from build123d import *

# Parameters (mm, degrees)
F1_DEPTH       = 6.22
F2_W           = 7
F2_H           = 1
F3_DEPTH       = 60.201
F4_R           = 0.1
F6_D           = 6.4
F6_CSINK_D     = 13.5
F6_CSINK_ANGLE = 90


with BuildPart() as f1:
    # F0 (on Front) → F1 (new body)
    with BuildSketch(Plane.XZ):
        with BuildLine():
            Line((-53.25, 0), (-0.5, 0))
            ThreePointArc((-0.5, 0), (-0.1464466094, 0.1464466094), (0, 0.5))
            Line((0, 0.5), (0, 59.7))
            ThreePointArc((0, 59.7), (-0.1464466094, 60.0535533906), (-0.5, 60.2))
            Line((-0.5, 60.2), (-53.25, 60.2))
            ThreePointArc((-53.25, 60.2), (-56.7855339059, 58.7355339059), (-58.25, 55.2))
            Line((-58.25, 55.2), (-58.25, 5))
            ThreePointArc((-58.25, 5), (-56.7855339059, 1.4644660941), (-53.25, 0))
        make_face()
    extrude(amount=F1_DEPTH)

    # F2 (on face) → F3 (cut, through all)
    with BuildSketch(Plane.XY.offset(60.2)):
        with Locations((-3.5, -0.5)):
            Rectangle(F2_W, F2_H)
    extrude(amount=-F3_DEPTH, mode=Mode.SUBTRACT)

    # F4
    f4_edges = [f1.edges().sort_by_distance(p)[0] for p in [
        (-26.875, -6.22, 60.2),
        (-30.125, 0, 60.2),
        (-7, 0, 30.1),
        (-3.75, -1, 60.2),
        (-7, -0.5, 60.2),
        (-7, -0.5, 0),
        (-7, -1, 30.1),
    ]]
    fillet(f4_edges, radius=F4_R)

    # F6 (through all)
    with Locations(Plane.XZ.offset(6.22)):
        with Locations((-30.25, 46.05), (-30.25, 14.15)):
            CounterSinkHole(F6_D / 2, F6_CSINK_D / 2, counter_sink_angle=F6_CSINK_ANGLE)


solid = f1.part
Read the model definition and answer for the solid it produces. Units are mm, in the model's axes. A direction names the side the tool comes from. Give positions to 0.01 mm unless a question says otherwise; leave off trailing zeros. Loops run counter-clockwise (first coordinate to the right, second up) from the corner with the lowest first, then second, coordinate; pieces in that order, holes last. Notation, with made-up numbers: M -37,53.25 L -28,53.25 A16 ccw -28,59.25 Z; hole C 76.5,46.5 d7. An arc over 180 degrees is marked long. Write each question's results on one line, items separated by ' | '.
1. Straight lines are drawn through the part: line 1 (Z direction, x = -30.25, y = -1.2); line 2 (X direction, y = -0.6, z = 14.15); line 3 (X direction, y = -1.4, z = 14.15). For each, find the intervals that lie inside material, in ascending order. Write a range as [from, to].
Values:
line 1: z = [0, 10.95], [17.35, 42.85], [49.25, 60.2] | line 2: x = [-58.25, -33.45], [-27.05, -7] | line 3: x = [-58.25, -33.45], [-27.05, 0]
2. Section A-A on z = 14.15 is taken. Give the vertices of the cut face in (x, y), plus the area to 3 significant figures.
Values:
outline: M -58.25,-6.12 A0.1 ccw -58.15,-6.22 L -37,-6.22 L -33.45,-2.67 L -33.45,0 L -58.15,0 A0.1 ccw -58.25,-0.1 Z; M -27.05,-2.67 L -23.5,-6.22 L -0.1,-6.22 A0.1 ccw 0,-6.12 L 0,-1.1 A0.1 ccw -0.1,-1 L -6.9,-1 A0.1 cw -7,-0.9 L -7,-0.1 A0.1 ccw -7.1,0 L -27.05,0 Z | area: 303 mm^2
3. Given pin 1 (3 mm diameter, centred on x = -27, z = 17, fed in from -Y); pin 2 (2 mm diameter, centred on x = -2, z = 17.5, fed in from +Y); pin 3 (0.6 mm diameter, centred on y = -0.5, z = 18, fed in from +X), each flat-ended and moving along its own axis, determine where each tip first touches the part or whether it passes through.
Values:
pin 1: stops at y = -5.29 | pin 2: stops at y = -1 | pin 3: stops at x = -7
4. Section C-C on z = 31 is taken. Give the vertices of the cut face in (x, y).
Values:
outline: M -58.25,-6.12 A0.1 ccw -58.15,-6.22 L -0.1,-6.22 A0.1 ccw 0,-6.12 L 0,-1.1 A0.1 ccw -0.1,-1 L -6.9,-1 A0.1 cw -7,-0.9 L -7,-0.1 A0.1 ccw -7.1,0 L -58.15,0 A0.1 ccw -58.25,-0.1 Z
5. Section B-B on x = -30.25 is taken. Give the vertices of the cut face in (y, z).
Values:
outline: M -6.22,0.1 A0.1 ccw -6.12,0 L -0.1,0 A0.1 ccw 0,0.1 L 0,10.95 L -2.67,10.95 L -6.22,7.4 Z; M -6.22,20.9 L -2.67,17.35 L 0,17.35 L 0,42.85 L -2.67,42.85 L -6.22,39.3 Z; M -6.22,52.8 L -2.67,49.25 L 0,49.25 L 0,60.1 A0.1 ccw -0.1,60.2 L -6.12,60.2 A0.1 ccw -6.22,60.1 Z
6. A tool of negligible diameter and unlimited length cuts with its end or side. For faces 1 (the face through (-27.053, -1.316, 14.291)), 2 (the face through (-4, -1, 31)), from which of +Z, -Z, +X, -X, +Y, -Y can it reach the whole face along a straight path? Write none if from no direction.
Values:
face 1: +Y, -Y | face 2: +Z, -Z, +X, +Y
7. The mould has two halves that part along Z. Classify faces 3 (the face through (-27, -3, 0)), 4 (the face through (-27.711, -1.316, 44.103)), 5 (the face through (0, -4, 30)): pulls with the +Z half, pulls with the -Z half, needs draft (parallel to the pull), parting line crosses it, or undercut.
Values:
face 3: pulls with the -Z half | face 4: undercut | face 5: needs draft
